Input: dimensioned drawing with shaded views. Units: mm. Origin: part minimum x, y, z. A direction names the side the tool comes from. Coordinates: 2 decimals unless noted, no trailing zeros. Loops run counter-clockwise (first coordinate to the right, second up) from the corner with the lowest first, then second, coordinate; pieces in that order, holes last.
Item 1: Reachability of the marked faces 1, 2 and 3 from +Z, -Z, +X, -X, +Y, -Y: full face, straight path, thin tool, end or side. Return the list, or none.
Item 2: Line query: probe 1 along X at (y, z) = (37, 25.5); probe 2 along Y at (x, z) = (5, 30); probe 3 along Z at (x, y) = (6.5, 25.5) (1 decimal). Output: solid intervals per line, ascending.
Item 3: Section query A-A, the plane x = 20.5. Return the cut outline in (y, z), then the cut area to 3 significant figures.
Item 4: Pull-direction query (X, two-part tool) for the marked faces 4, 5 and 6; classes: +X half, -X half, draft (parallel to the pull), parting line (faces both ways), or undercut.
Item 5: Section query B-B, the plane z = 30. Return the cut outline in (x, y).
Item 6: Pin query (flat end, axial travel): pin 1 Ø19 at (x, y) = (17.5, 7) entering from +Z (1 decimal); pin 2 Ø9 at (y, z) = (27, 37.5) entering from -X; pin 3 Ø5 at (x, z) = (28.5, 26.5) entering from +Y (1 decimal). Return the tip coordinate at first contact, or that it passes through.
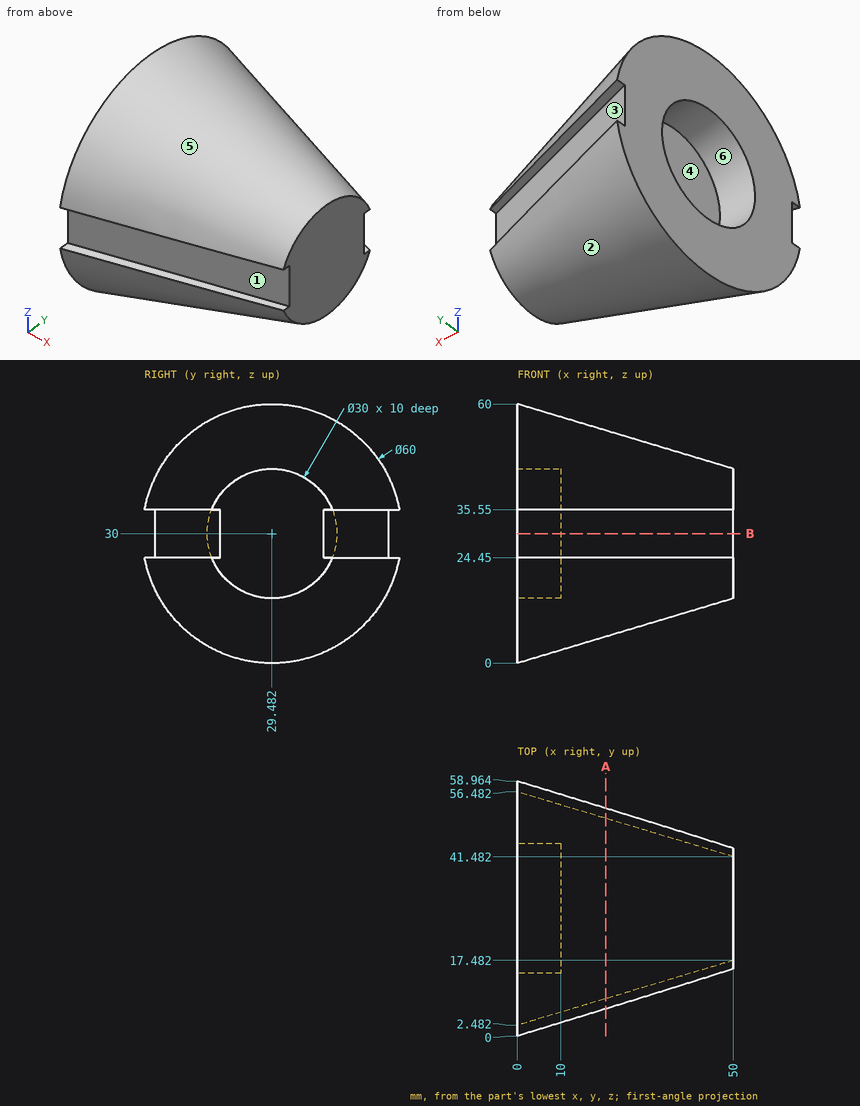
Verdict:
1. face 1: +X, -Y
1. face 2: -Z, +X
1. face 3: +X, +Y
2. probe 1: x = 10 to 50
2. probe 2: y = 3.98 to 14.48, 44.48 to 54.98
2. probe 3: z = 2.2 to 15.5, 44.5 to 57.8
3. outline: (6.29, 24.45) arc R23.85 ccw to (52.68, 24.45) - (50.33, 24.45) - (50.33, 35.55) - (52.68, 35.55) arc R23.85 ccw to (6.29, 35.55) - (8.63, 35.55) - (8.63, 24.45) - close
3. area: 1,730 mm2
4. face 4: -X half
4. face 5: +X half
4. face 6: draft
5. outline: (0, 2.48) - (50, 17.48) - (50, 41.48) - (0, 56.48) - (0, 44.48) - (10, 44.48) - (10, 14.48) - (0, 14.48) - close
6. pin 1: stops at z = 52
6. pin 2: stops at x = 10
6. pin 3: stops at y = 50.6
